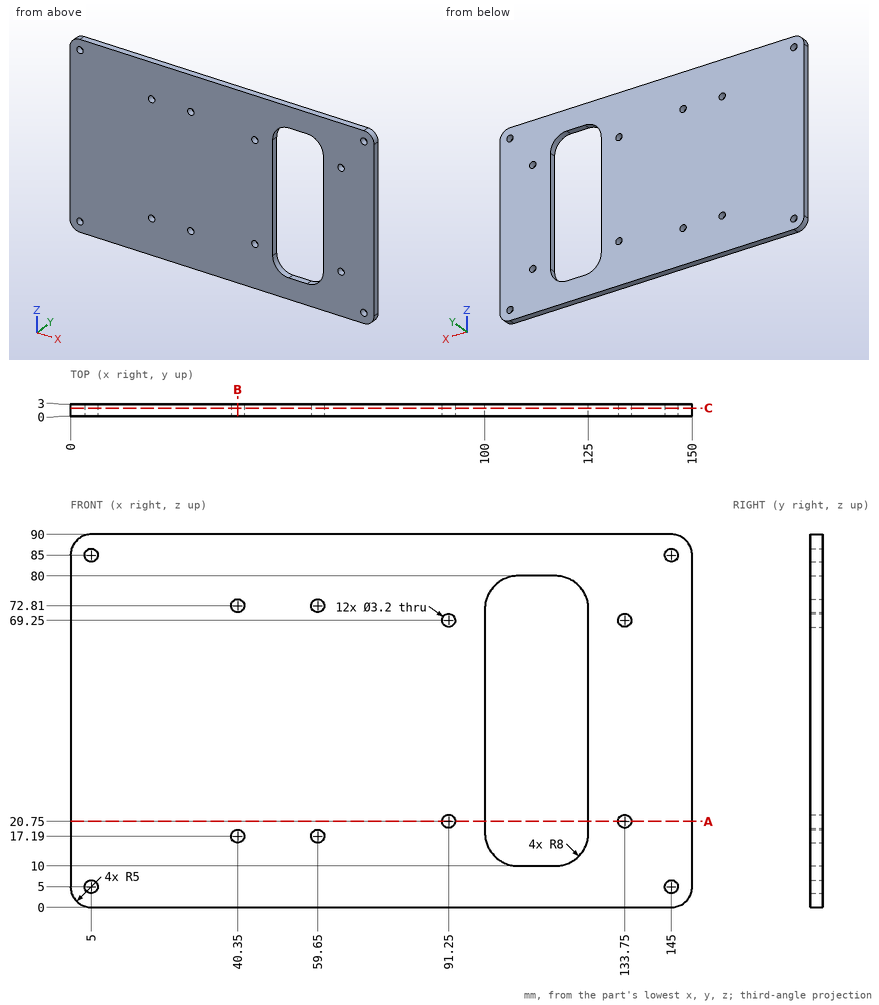
Here's the drawing with two shaded views (mm, measured from the low corner). I have some questions. Round coordinates to 2 decimals unless told otherwise and drop trailing zeros. Loops run counter-clockwise (first coordinate to the right, second up) from the corner with the lowest first, then second, coordinate; pieces in that order, holes last.
Item 1: Please list where these lines run through material, in increasing order: L1, parallel to X at y = 1.5, z = 85; L2, parallel to Z at x = 91.25, y = 1.55; L3, parallel to X at y = 0.35, z = 69.5.
Item 2: Will these pins go through, and if not, where does the flat tip stop? pin 1 Ø5 at (x, z) = (5, 5) entering from +Y; pin 2 Ø1.9 at (x, z) = (40.35, 72.81) entering from -Y.
Item 3: Suppose I cut it at A-A, the plane z = 20.75. Write out the boundary of the cut face in (x, y), then the cut area to 3 significant figures.
Item 4: Suppose I cut it at C-C, the plane y = 2. State how many separate pieces and enclosed holes the cut face has, then the cut area to 3 significant figures.
Item 5: Suppose I cut it at B-B, the plane x = 40.35. Write out the boundary of the cut face in (y, z).
Reported:
1. L1: x = 0 to 3.4, 6.6 to 143.4, 146.6 to 150
1. L2: z = 0 to 19.15, 22.35 to 67.65, 70.85 to 90
1. L3: x = 0 to 89.67, 92.83 to 100, 125 to 132.17, 135.33 to 150
2. pin 1: stops at y = 3
2. pin 2: passes through
3. outline: (0, 0) - (89.65, 0) - (89.65, 3) - (0, 3) - close; (92.85, 0) - (100, 0) - (100, 3) - (92.85, 3) - close; (125, 0) - (132.15, 0) - (132.15, 3) - (125, 3) - close; (135.35, 0) - (150, 0) - (150, 3) - (135.35, 3) - close
3. area: 356 mm2
4. separate pieces: 1
4. enclosed holes: 13
4. area: 11,700 mm2
5. outline: (0, 0) - (3, 0) - (3, 15.59) - (0, 15.59) - close; (0, 18.79) - (3, 18.79) - (3, 71.21) - (0, 71.21) - close; (0, 74.41) - (3, 74.41) - (3, 90) - (0, 90) - close
